Input: part model. Units: mm. Frame: model coordinates. Face numbers are marked on the shaded views. A direction names the side the tool comes from. Round coordinates to 2 decimals unless told otherwise and drop trailing zeros. Loops run counter-clockwise (first coordinate to the right, second up) from the corner with the lowest first, then second, coordinate; pieces in that order, holes last. Notation, with made-up numbers: M 33.5,85 L 50.5,85 A9 cw 50.5,96 Z; hole C -23.75,-30 d11. An arc over 180 degrees is marked long. Use one line per item in the form item = value. Start each with the question number.
Q1. Section query B-B, the plane y = 18.5. Output: boundary loops of the cut face in (x, z).
Q2. Section query C-C, the plane x = -9. Output: boundary loops of the cut face in (y, z).
Q3. First-contact query: P1, Ø3, axis at x = -9.5, y = 20, coming from the +Z side; P2, Ø5, axis at x = -5, z = 7.5, coming from the -Y side. Flat tips, straight axial feed; report the tip coordinate or a pass-through.
Q4. Mould query, pull axis X, two halves, no side actions, for the marked faces 3, 4, 5 and 6. Classes: pulls with the +X half, pulls with the -X half, needs draft (parallel to the pull), parting line crosses it, or undercut.
Q5. Ray query, line 1 along X through (y, z) = (21, 12.75); line 2 along Z through (x, y) = (4.5, 9.5); line 3 along Y through (x, z) = (-8.5, 10). Return the intervals inside material, ascending.
Q6. Access query for the marked faces 1 and 2. Directions: +Z, -Z, +X, -X, +Y, -Y. A direction counts if a zero-diameter tool reaches every point of the face in a straight line with its end or side. Return the directions, or none.
Q7. Section query A-A, the plane z = 4.25. Output: boundary loops of the cut face in (x, y), and give its area (3 significant figures).
Q8. Section query D-D, the plane z = 1.75. Output: boundary loops of the cut face in (x, y), and give its area (3 significant figures).
```python
from build123d import *

# Parameters (mm, degrees)
F0_W          = 36
F0_H          = 45
F1_DEPTH      = 3
F3_DEPTH      = 3
F5_DEPTH      = 10
F5_DEPTH_BACK = 3
F6_R          = 2.3
F7_R          = 5


with BuildPart() as f1:
    # F0 (on Top) → F1 (new body)
    with BuildSketch(Plane.XY):
        Rectangle(F0_W, F0_H)
    extrude(amount=F1_DEPTH)

    # F2 (on face) → F3 (cut)
    with BuildSketch(Plane.XY.offset(3)):
        with BuildLine():
            Line((-7, -22.5), (-7, -4.5))
            ThreePointArc((-7, -4.5), (-8.9668645083, -2.500274509), (-10.9989020392, -4.4337381126))
            Line((-10.9989020392, -4.4337381126), (-10.9989020392, -4.5662618874))
            Line((-10.9989020392, -4.5662618874), (-10.9989020392, -22.5))
            Line((-10.9989020392, -22.5), (-7, -22.5))
        make_face()
        with BuildLine():
            Line((7, -4.5), (7, -22.5))
            Line((7, -22.5), (10.9989020392, -22.5))
            Line((10.9989020392, -22.5), (10.9989020392, -4.5662618874))
            Line((10.9989020392, -4.5662618874), (10.9989020392, -4.4337381126))
            ThreePointArc((10.9989020392, -4.4337381126), (8.9668645083, -2.500274509), (7, -4.5))
        make_face()
    extrude(amount=-F3_DEPTH, mode=Mode.SUBTRACT)

    # F4 (on face) → F5 (join, two sides)
    with BuildSketch(Plane.XY.offset(3)) as f5_sk:
        Polygon((18, -22.5), (20.9999997169, -22.5), (20.9999997169, 25.4999997169), (-20.9999997169, 25.4999997169), (-20.9999997169, -22.5), (-18, -22.5), (-18, 22.5), (18, 22.5), align=None)
    extrude(amount=F5_DEPTH)
    extrude(f5_sk.sketch, amount=-F5_DEPTH_BACK)

    # F6
    f6_edges = [f1.edges().sort_by_distance(p)[0] for p in [
        (-10.998902, -22.5, 1.5),
        (-7, -22.5, 1.5),
        (7, -22.5, 1.5),
        (10.998902, -22.5, 1.5),
    ]]
    fillet(f6_edges, radius=F6_R)

    # F7
    f7_edges = [f1.edges().sort_by_distance(p)[0] for p in [
        (-19.5, -22.5, 13),
        (19.5, -22.5, 13),
    ]]
    fillet(f7_edges, radius=F7_R)


solid = f1.part
```
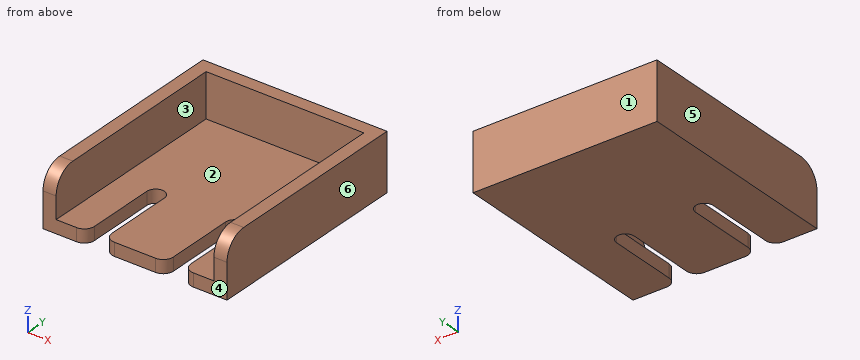
Results found:
q1.outline = M -21,0 L 21,0 L 21,13 L 18,13 L 18,3 L -18,3 L -18,13 L -21,13 Z
q2.outline = M -2.5,0 L 25.5,0 L 25.5,13 L 22.5,13 L 22.5,3 L -2.5,3 Z
q3.P1 = 3
q3.P2 = 22.5
q4.face_3 = undercut
q4.face_4 = needs draft
q4.face_5 = pulls with the -X half
q4.face_6 = pulls with the +X half
q5.line_1 = -21 to -18, 18 to 21
q5.line_2 = 0 to 3
q5.line_3 = 22.5 to 25.5
q6.face_1 = +Z, -Z, +X, -X, +Y
q6.face_2 = +Z, -Y
q7.outline = M -21,-22.5 L -18,-22.5 L -18,22.5 L 18,22.5 L 18,-22.5 L 21,-22.5 L 21,25.5 L -21,25.5 Z
q7.area = 396 mm²
q8.outline = M -21,-22.5 L -13.3,-22.5 A2.3 ccw -11,-20.2 L -11,-4.43 A2 cw -7,-4.5 L -7,-20.2 A2.3 ccw -4.7,-22.5 L 4.7,-22.5 A2.3 ccw 7,-20.2 L 7,-4.5 A2 cw 11,-4.43 L 11,-20.2 A2.3 ccw 13.3,-22.5 L 21,-22.5 L 21,25.5 L -21,25.5 Z
q8.area = 1,850 mm²
